Source: CAD feature listing. Evaluate the final solid. Frame: model axes, mm. Face numbers are marked on the shaded views. A direction names the side the tool comes from. Round coordinates to 2 decimals unless told otherwise and drop trailing zeros. Loops run counter-clockwise (first coordinate to the right, second up) from the corner with the lowest first, then second, coordinate; pieces in that order, holes last.
(1) Mould query, pull axis X, two halves, no side actions, for the marked faces 1, 2, 3 and 4. Classes: pulls with the +X half, pulls with the -X half, needs draft (parallel to the pull), parting line crosses it, or undercut.
(2) Section C-C, the plane y = 35.75. Return the cut outline in (x, z).
(3) Section A-A, the plane y = -0.25. Return the cut outline in (x, z), plus the area to 3 significant figures.
(4) Section B-B, the plane x = -18. Return the cut outline in (y, z), plus the area to 3 significant figures.
(5) Section D-D, the plane z = -1.5. Return the cut outline in (x, y), plus the area to 3 significant figures.
(6) Material intervals for probe 1 along Y at (x, z) = (-16.5, -4.3); probe 2 along Z at (x, y) = (1, 7.5); probe 3 along X at (y, z) = (35, -1), sorted ascending.
(7) Set-up query: the marked faces 5, 6 and 7. Return all of +Z, -Z, +X, -X, +Y, -Y with unobstructed straight access to the full face (end or side cutting, diameter ignored); none if empty.
(8) First-contact query: pin 1 Ø14.5 at (x, z) = (0, 18.5) entering from -Y; pin 2 Ø8 at (x, y) = (16.5, -0.25) entering from +Z; pin 3 Ø9 at (x, z) = (-2.5, 9) entering from +Y; pin 4 Ø4.5 at (y, z) = (-2.5, 8.5) entering from -X. Flat tips, straight axial feed; report the tip coordinate or a pass-through.
```python
from build123d import *

# Parameters (mm, degrees)
F0_W     = 48
F0_H     = 51
F1_DEPTH = 6
F2_R     = 5
F3_D     = 5
F4_R     = 5.5
F5_DEPTH = 15


with BuildPart() as f1:
    # F0 (on Top) → F1 (new body)
    with BuildSketch(Plane.XY):
        with Locations((0, 17.75)):
            Rectangle(F0_W, F0_H)
    extrude(amount=-F1_DEPTH)

    # F2
    f2_edges = [f1.edges().sort_by_distance(p)[0] for p in [
        (24, -7.75, -3),
        (24, 43.25, -3),
        (-24, 43.25, -3),
        (-24, -7.75, -3),
    ]]
    fillet(f2_edges, radius=F2_R)

    # F3 (through all)
    with Locations(Plane.XY):
        with Locations((16.5, -0.25), (-16.5, -0.25), (16.5, 35.75), (-16.5, 35.75)):
            Hole(F3_D / 2)

    # F4 (on face) → F5 (join)
    with BuildSketch(Plane.XZ.offset(7.75)):
        with BuildLine():
            Line((9, 0), (9, 18.5))
            ThreePointArc((9, 18.5), (0, 27.5), (-9, 18.5))
            Line((-9, 18.5), (-9, 0))
            Line((-9, 0), (9, 0))
        make_face()
        with Locations((0, 18.5)):
            Circle(F4_R, mode=Mode.SUBTRACT)
    extrude(amount=-F5_DEPTH)


solid = f1.part
```
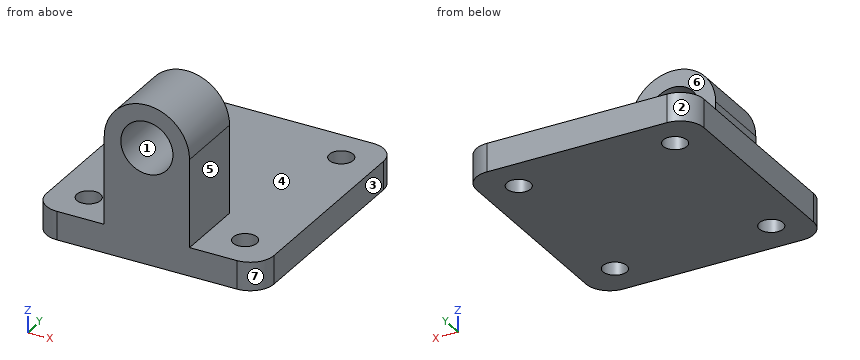
Output values:
1. face 1: undercut
1. face 2: pulls with the -X half
1. face 3: pulls with the +X half
1. face 4: needs draft
2. outline: (-24, -6) - (-19, -6) - (-19, 0) - (-24, 0) - close; (-14, -6) - (14, -6) - (14, 0) - (-14, 0) - close; (19, -6) - (24, -6) - (24, 0) - (19, 0) - close
3. outline: (-24, -6) - (-19, -6) - (-19, 0) - (-24, 0) - close; (-14, -6) - (14, -6) - (14, 0) - (9, 0) - (9, 18.5) arc R9 ccw to (-9, 18.5) - (-9, 0) - (-14, 0) - close; (19, -6) - (24, -6) - (24, 0) - (19, 0) - close; hole circle Ø11 at (0, 18.5)
3. area: 593 mm2
4. outline: (-7.75, -6) - (-2.25, -6) - (-2.25, 0) - (-7.75, 0) - close; (1.75, -6) - (33.75, -6) - (33.75, 0) - (1.75, 0) - close; (37.75, -6) - (43.25, -6) - (43.25, 0) - (37.75, 0) - close
4. area: 258 mm2
5. outline: (-24, -2.75) arc R5 ccw to (-19, -7.75) - (19, -7.75) arc R5 ccw to (24, -2.75) - (24, 38.25) arc R5 ccw to (19, 43.25) - (-19, 43.25) arc R5 ccw to (-24, 38.25) - close; hole circle Ø5 at (-16.5, -0.25); hole circle Ø5 at (-16.5, 35.75); hole circle Ø5 at (16.5, -0.25); hole circle Ø5 at (16.5, 35.75)
5. area: 2,350 mm2
6. probe 1: y = -7.75 to -2.75, 2.25 to 33.25, 38.25 to 43.25
6. probe 2: z = -6 to 0
6. probe 3: x = -24 to -18.88, -14.12 to 14.12, 18.88 to 24
7. face 5: +Z, +X, +Y, -Y
7. face 6: +Z, +X, -X, +Y
7. face 7: +Z, -Z, +X, -Y
8. pin 1: stops at y = -7.75
8. pin 2: stops at z = 0
8. pin 3: stops at y = 7.25
8. pin 4: stops at x = -9
